Autodesk Inventor part; units mm, degrees
ref_plane "YZ Plane" through (0, 0, 0) normal (1, 0, 0) x (0, 1, 0)
ref_plane "XZ Plane" through (0, 0, 0) normal (0, 1, 0) x (-1, 0, 0)
ref_plane "XY Plane" through (0, 0, 0) normal (0, 0, 1) x (1, 0, 0)
sketch "Sketch1" plane through (0, 0, 0) normal (0, 0, 1) x (1, 0, 0)
  line L0 (-12.1708, 16.0073) -> (13.2292, 16.0073)
  line L1 (13.2292, 16.0073) -> (13.2292, -34.7927)
  line L2 (13.2292, -34.7927) -> (-12.1708, -34.7927)
  line L3 (-12.1708, -34.7927) -> (-12.1708, 16.0073)
  line L4 (11.9592, 14.7373) -> (-10.9008, 14.7373)
  line L5 (-10.9008, 14.7373) -> (-10.9008, -33.5227)
  line L6 (-10.9008, -33.5227) -> (11.9592, -33.5227)
  line L7 (11.9592, -33.5227) -> (11.9592, 14.7373)
  point P0 (0, 0)
  dimension "d0" = 25.4
  dimension "d1" = 50.8
  dimension "d2" = 1.27
extrude "Extrusion1" add sketch "Sketch1" along normal blind 381
sketch "Sketch2" plane through (-12.1708, 16.0073, 0) normal (0, 1, 0) x (1, 0, 0)
  circle A0 centre (12.7, -12.7) radius 1.7272
  line L0 (25.4, 0) -> (0, 0)
  line L1 (0, 0) -> (0, -381)
  point P0 (12.1708, 0)
  dimension "d5" = 3.4544
  dimension "d6" = 12.7
  dimension "d7" = 12.7
extrude "Extrusion2" cut sketch "Sketch2" against normal through all
pattern_linear "Rectangular Pattern1" count 38 spacing 25.4 along (0, 0, 1) of "Extrusion2"
sketch "Sketch5" plane through (13.2292, -34.7927, 0) normal (1, 0, 0) x (0, 0, -1)
  circle A0 centre (-348.9452, 25.4) radius 14.2875
  line L0 (-381, 0) -> (-381, 50.8)
  line L1 (0, 50.8) -> (-381, 50.8)
  circle A1 centre (-231.4448, 25.4) radius 14.2875
  circle A2 centre (-35.4076, 25.4) radius 14.2875
  point P0 (0, 34.7927)
  dimension "d46" = 28.575
  dimension "d47" = 32.0548
  dimension "d48" = 25.4
  dimension "d49" = 28.575
  dimension "d50" = 149.5552
  dimension "d51" = 25.4
  dimension "d52" = 28.575
  dimension "d53" = 345.5924
  dimension "d54" = 25.4
extrude "Extrusion5" cut sketch "Sketch5" against normal through all
equation "\"d3\" = d13"
equation "\"d10\" = d14"
equation "\"d13\" = 381"
equation "\"d14\" = d13"
equation "\"d32\" = 101.6"
properties part number "VersaFrame 28in"
Here's how the part is built. I have some questions about the finished solid (model axes, mm). A direction names the side the tool comes from. Give positions to 0.01 mm unless a question says otherwise; leave off trailing zeros. Loops run counter-clockwise (first coordinate to the right, second up) from the corner with the lowest first, then second, coordinate; pieces in that order, holes last. Notation, with made-up numbers: (46.5, 47) -> (83.5, 47) arc R23 ccw to (83.5, 66) -> close; hole circle Ø1 at (5, 64). An arc over 180 degrees is marked (long way). Answer as a JSON object with one key per item and string values. Group by question number.
Item 1: Imagine slicing it at B-B on y = -5. Give the number of separate pieces and of enclosed holes in the cut face, then the cut area to 3 significant figures.
Item 2: Thinking about a two-plate mould opening in Y: for faces 3 (the flat face through (1, -34.793, 188)), 4 (the flat face through (-12, -9, 0)), 5 (the cylindrical face through (12.603, -14.865, 335.747)), which applies, pulls with the +Y half, pulls with the -Y half, needs draft (parallel to the pull), parting line crosses it, or undercut?
Item 3: Imagine slicing it at A-A on z = 199. Write out the boundary of the cut face in (x, y).
Item 4: Will these pins go through, and if not, where does the flat tip stop? pin 1 (3 mm diameter, centred on x = 0.53, z = 266.7, fed in from -Y); pin 2 (4.5 mm diameter, centred on x = 0.53, z = 342.9, fed in from -Y).
Item 5: I need wall thicknesses on L1, parallel to Z at x = -11, y = -9; L2, parallel to X at y = 11, z = 360; L3, parallel to Y at x = 4, z = 274. Which ranges of each line are inside material? Lowest first, please.
Item 6: On a 3-axis mill with a long thin cutter (end or side, diameter ignored), from which of +Z, -Z, +X, -X, +Y, -Y can I reach the whole of each face in a straight line? I mean faces 1 (the flat face through (0, 16.007, 188)), 2 (the flat face through (11.959, -10, 188)). Say none if no direction works.
Answer list:
{
 "1": {"separate pieces": "8", "enclosed holes": "0", "area": "761 mm2"},
 "2": {"face 3": "pulls with the -Y half", "face 4": "needs draft", "face 5": "undercut"},
 "3": {"outline": "(-12.17, -34.79) -> (13.23, -34.79) -> (13.23, 16.01) -> (-12.17, 16.01) -> close; hole (-10.9, -33.52) -> (11.96, -33.52) -> (11.96, 14.74) -> (-10.9, 14.74) -> close"},
 "4": {"pin 1": "passes through", "pin 2": "stops at y = -34.79"},
 "5": {"L1": "z = 0 to 21.13, 49.69 to 217.16, 245.73 to 334.66, 363.23 to 381", "L2": "x = -12.17 to -10.9, 11.96 to 13.23", "L3": "y = -34.79 to -33.52, 14.74 to 16.01"},
 "6": {"face 1": "+Z, -Z, +X, -X, +Y", "face 2": "+Z, -Z"}
}
